Geometry check sheet. Reference: the model listing, model coordinates, mm. A direction names the side the tool comes from. Coordinates: 2 decimals unless noted, no trailing zeros. Loops run counter-clockwise (first coordinate to the right, second up) from the corner with the lowest first, then second, coordinate; pieces in that order, holes last.
from build123d import *

# Parameters (mm, degrees)
SKETCH_1_R          = 9.975
EXTRUDE_1_DEPTH     = 40
SKETCH_5_R          = 9.975
F_16MM_DEPTH        = 16
SKETCH_6_R          = 9.45
EXTRUDE_1_2_DEPTH   = 1
SKETCH_7_R          = 9.975
EXTRUDE_4_DEPTH     = 45
SKETCH_8_R          = 9.45
EXTRUDE_2_DEPTH     = 1
SKETCH_9_R          = 9.975
EXTRUDE_6_DEPTH     = 1
CUT_EXTRUDE_1_DEPTH = 8


with BuildPart() as part:
    # 草图1 → Extrude 1 (new body)
    with BuildSketch(Plane(origin=(0, 0, 0), x_dir=(1, 0, 0), z_dir=(0, 1, 0))):
        with Locations(Location((5.9, 0, 0), (0, 0, 270))):
            Circle(SKETCH_1_R)
    extrude(amount=EXTRUDE_1_DEPTH)

    # 草图5 → 16mm 铰链间距 (add)
    with BuildSketch(Plane(origin=(0, 40, 0), x_dir=(1, 0, 0), z_dir=(0, 1, 0))):
        with Locations(Location((5.9, 0, 0), (0, 0, 270))):
            Circle(SKETCH_5_R)
    extrude(amount=F_16MM_DEPTH)

    # 草图6 → Extrude 1 2 (add)
    with BuildSketch(Plane(origin=(0, 56, 0), x_dir=(1, 0, 0), z_dir=(0, 1, 0))):
        with Locations(Location((5.9, 0, 0), (0, 0, 270))):
            Circle(SKETCH_6_R)
    extrude(amount=EXTRUDE_1_2_DEPTH)

    # 草图7 → 凸台-拉伸4 (add)
    with BuildSketch(Plane(origin=(0, 57, 0), x_dir=(1, 0, 0), z_dir=(0, 1, 0))):
        with Locations(Location((5.9, 0, 0), (0, 0, 270))):
            Circle(SKETCH_7_R)
    extrude(amount=EXTRUDE_4_DEPTH)

    # 草图8 → 卡簧2 (add)
    with BuildSketch(Plane(origin=(0, 102, 0), x_dir=(1, 0, 0), z_dir=(0, 1, 0))):
        with Locations(Location((5.9, 0, 0), (0, 0, 270))):
            Circle(SKETCH_8_R)
    extrude(amount=EXTRUDE_2_DEPTH)

    # 草图9 → 凸台-拉伸6 (add)
    with BuildSketch(Plane(origin=(0, 103, 0), x_dir=(1, 0, 0), z_dir=(0, 1, 0))):
        with Locations(Location((5.9, 0, 0), (0, 0, 270))):
            Circle(SKETCH_9_R)
    extrude(amount=EXTRUDE_6_DEPTH)

    # 草图10 → 切除-拉伸1 (cut)
    with BuildSketch(Plane.XY.offset(9.975)):
        Polygon((8.65, 9.58771324), (5.9, 11.175426481), (3.15, 9.58771324), (3.15, 6.41228676), (5.9, 4.824573519), (8.65, 6.41228676), align=None)
    cut_extrude_1 = extrude(amount=-CUT_EXTRUDE_1_DEPTH, mode=Mode.SUBTRACT)

    # 镜向2: 切除-拉伸1 across plane
    add(cut_extrude_1.mirror(Plane(origin=(0, 20, 0), x_dir=(0, 0, 1), z_dir=(0, -1, 0))), mode=Mode.SUBTRACT)


solid = part.part
(1) Sectioned sample at A-A on x = 2. Record the cut outline in (y, z).
Findings:
outline: (0, -9.18) - (56, -9.18) - (56, -8.61) - (57, -8.61) - (57, -9.18) - (102, -9.18) - (102, -8.61) - (103, -8.61) - (103, -9.18) - (104, -9.18) - (104, 9.18) - (103, 9.18) - (103, 8.61) - (102, 8.61) - (102, 9.18) - (57, 9.18) - (57, 8.61) - (56, 8.61) - (56, 9.18) - (0, 9.18) - close
(2) Scan lines: L1, parallel to Y at x = 11, z = 8.5; L2, parallel to X at y = 88, z = -0.5; L3, parallel to Y at x = 7.75, z = 2.75. Record each from-to range of solid material in increasing order.
Findings:
L1: y = 0 to 56, 57 to 102, 103 to 104
L2: x = -4.06 to 15.86
L3: y = 0 to 5.89, 10.11 to 29.89, 34.11 to 104
(3) Access from +Z, -Z, +X, -X, +Y, -Y to the whole of each face (thin tool, end or side, straight path). Record for faces 3 (the flat face through (4.506, 34.37, 6.031)), 4 (the flat face through (-3, 57, 4)), 5 (the cylindrical face through (-3.84, 79.18, -2.16)).
Findings:
face 3: +Z
face 4: none
face 5: +Y, -Y
(4) Gauge pin test, flat ends, axial feed: pin 1 Ø3.5 at (y, z) = (7.5, 5) entering from -X; pin 2 Ø6 at (x, y) = (0, 91) entering from +Z; pin 3 Ø2.5 at (y, z) = (7.5, 5) entering from +X; pin 4 Ø4 at (x, z) = (10.5, 3.5) entering from -Y. Record the tip position at first contact, or that the pin passes through.
Findings:
pin 1: stops at x = -3.53
pin 2: stops at z = 9.54
pin 3: stops at x = 15.14
pin 4: stops at y = 0
(5) Sectioned sample at D-D on y = 54. Record the cut outline in (x, z) (3 decimals), and give its area (3 significant figures).
Findings:
outline: circle Ø19.95 at (5.9, 0)
area: 313 mm2
(6) Sectioned sample at B-B on z = -6.75. Record the cut outline in (x, y).
Findings:
outline: (-1.44, 0) - (13.24, 0) - (13.24, 56) - (12.51, 56) - (12.51, 57) - (13.24, 57) - (13.24, 102) - (12.51, 102) - (12.51, 103) - (13.24, 103) - (13.24, 104) - (-1.44, 104) - (-1.44, 103) - (-0.71, 103) - (-0.71, 102) - (-1.44, 102) - (-1.44, 57) - (-0.71, 57) - (-0.71, 56) - (-1.44, 56) - close
(7) Draft check along Y on faces 1 (the flat face through (7.294, 29.63, 6.031)), 2 (the cylindrical face through (-3.84, 103.49, -2.16)). Enter one of: +Y half, -Y half, draft (parallel to the pull), parting line (faces both ways), or undercut.
Findings:
face 1: undercut
face 2: draft
(8) Sectioned sample at C-C on z = 6.25. State how many separate pieces and enclosed holes the cut face has, and give its area (3 significant figures).
Findings:
separate pieces: 1
enclosed holes: 2
area: 1,560 mm2
